Input: part model. Units: mm. Frame: model coordinates. A direction names the side the tool comes from. Give positions to 0.01 mm unless a question says otherwise; leave off trailing zeros. Write each loop counter-clockwise with the first axis right and the second up, starting at its lowest first coordinate (ties: lowest second). Pieces come first, ordered by that corner, then holes. Notation, with made-up numbers: (54.5, 64.25) - (68.5, 64.25) arc R12 cw to (68.5, 78.25) - close; hole circle Ø5 at (30.25, -25). An arc over 180 degrees is marked (long way). Use a Markdown table: item, result. Add a question column.
1. Pin query (flat end, axial travel): pin 1 (2 mm diameter, centred on y = 0, z = -2, fed in from -X); pin 2 (1.2 mm diameter, centred on y = -2, z = -1, fed in from +X); pin 3 (1.5 mm diameter, centred on y = -5.5, z = 3, fed in from +X). Return the tip coordinate at first contact, or that it passes through.
2. Section query D-D, the plane z = 20.75. Return loops of the section in (x, y) (3 decimals), plus the area to 3 significant figures.
3. Section query A-A, the plane y = 0. Count the separate pieces of the cut face and the enclosed holes in it, plus the area to 3 significant figures.
4. Section query B-B, the plane z = 3. Return loops of the section in (x, y) (3 decimals), plus the area to 3 significant figures.
5. Mould query, pull axis X, two halves, no side actions, for faces 1 (the flat face through (-4, -0.1, -4.5)), 2 (the flat face through (0, -8.85, -2)), 3 (the flat face through (0, 7, 1)). Classes: released by +X, released by -X, zero draft, split by the parting line, or undercut.
6. Set-up query: faces 4 (the flat face through (0, 8.85, -2)), 5 (the flat face through (-0.07, 8.04, 6.99)), 6 (the flat face through (-3, 0, 1)). Return all of +Z, -Z, +X, -X, +Y, -Y with unobstructed straight access to the full face (end or side cutting, diameter ignored); none if empty.
7. Section query C-C, the plane x = 0. Return loops of the section in (y, z), plus the area to 3 significant figures.
8. Material intervals for probe 1 along Z at (x, y) = (11.25, 1.25); probe 2 along X at (y, z) = (-1.25, 20); probe 3 along Y at (x, z) = (1.75, 17), sorted ascending.
```python
from build123d import *

# Parameters (mm, degrees)
CROQUIS1_R              = 12.5
SALIENTE_EXTRUIR1_DEPTH = 24
CROQUIS2_W              = 9.3
CROQUIS2_H              = 18
CORTAR_EXTRUIR1_DEPTH   = 18
CROQUIS3_W              = 9
CROQUIS3_H              = 17.7
SALIENTE_EXTRUIR2_DEPTH = 5
CHAFL_N1_SIZE           = 1
CHAFL_N2_SIZE           = 1
CROQUIS4_R              = 2
CORTAR_EXTRUIR2_DEPTH   = 34.963215395
CHAFL_N3_SIZE           = 1
CROQUIS5_W              = 6
CROQUIS5_H              = 14
CORTAR_EXTRUIR3_DEPTH   = 26.228951623
CHAFL_N4_SIZE           = 1.95


with BuildPart() as part:
    # Croquis1 → Saliente-Extruir1 (new body)
    with BuildSketch(Plane.XY):
        Circle(CROQUIS1_R)
    extrude(amount=SALIENTE_EXTRUIR1_DEPTH)

    # Croquis2 → Cortar-Extruir1 (cut)
    with BuildSketch(Plane.XY.offset(24)):
        Rectangle(CROQUIS2_W, CROQUIS2_H)
    extrude(amount=-CORTAR_EXTRUIR1_DEPTH, mode=Mode.SUBTRACT)

    # Croquis3 → Saliente-Extruir2 (add)
    with BuildSketch(Plane(origin=(0, 0, 0), x_dir=(-1, 0, 0), z_dir=(0, 0, -1))):
        Rectangle(CROQUIS3_W, CROQUIS3_H)
    extrude(amount=SALIENTE_EXTRUIR2_DEPTH)

    # Chaflán1
    chafl_n1_edges = [part.edges().sort_by_distance(p)[0] for p in [
        (-4.5, 0, -5),
        (0, 8.85, -5),
        (4.5, 0, -5),
        (0, -8.85, -5),
    ]]
    chamfer(chafl_n1_edges, length=CHAFL_N1_SIZE)

    # Chaflán2
    chafl_n2_edges = [part.edges().sort_by_distance(p)[0] for p in [
        (-12.5, 0, 0),
    ]]
    chamfer(chafl_n2_edges, length=CHAFL_N2_SIZE)

    # Croquis4 → Cortar-Extruir2 (cut, through all)
    with BuildSketch(Plane.XY.offset(24)):
        with Locations((-7.875, 0)):
            Circle(CROQUIS4_R)
        with Locations((7.875, 0)):
            Circle(CROQUIS4_R)
    extrude(amount=-CORTAR_EXTRUIR2_DEPTH, mode=Mode.SUBTRACT)

    # Chaflán3
    chafl_n3_edges = [part.edges().sort_by_distance(p)[0] for p in [
        (-12.5, 0, 24),
    ]]
    chamfer(chafl_n3_edges, length=CHAFL_N3_SIZE)

    # Croquis5 → Cortar-Extruir3 (cut, through all)
    with BuildSketch(Plane.XY.offset(6)):
        Rectangle(CROQUIS5_W, CROQUIS5_H)
    extrude(amount=-CORTAR_EXTRUIR3_DEPTH, mode=Mode.SUBTRACT)

    # Chaflán4
    # the kernel refuses this chamfer: 1.95 mm, written as the material it adds along each edge
    with BuildSketch(Plane(origin=(4.65, 9, 6), x_dir=(0.02749587661058626, 0, 0.9996219169112968), z_dir=(0, -1, 0))) as chafl_n4_piece_1_section:
        Polygon((CHAFL_N4_SIZE * 0.999621916911, CHAFL_N4_SIZE * 0.0274958766106), (-CHAFL_N4_SIZE * 0.0274958766106, CHAFL_N4_SIZE * 0.999621916911), (0, 0), align=None)
    chafl_n4_piece_1 = extrude(amount=18, mode=Mode.PRIVATE)
    chafl_n4_piece_1 = split(chafl_n4_piece_1, bisect_by=Plane(origin=(3, 8, 6.663333333), z_dir=(1, 0, 0)), keep=Keep.TOP, mode=Mode.PRIVATE)
    add(chafl_n4_piece_1)
    with BuildSketch(Plane(origin=(4.65, 9, 6), x_dir=(0.02749587661058626, 0, 0.9996219169112968), z_dir=(0, -1, 0))) as chafl_n4_piece_2_section:
        Polygon((CHAFL_N4_SIZE * 0.999621916911, CHAFL_N4_SIZE * 0.0274958766106), (-CHAFL_N4_SIZE * 0.0274958766106, CHAFL_N4_SIZE * 0.999621916911), (0, 0), align=None)
    chafl_n4_piece_2 = extrude(amount=23.014781827, mode=Mode.PRIVATE)
    chafl_n4_piece_2 = split(chafl_n4_piece_2, bisect_by=Plane(origin=(2.9, 7, 6.1), z_dir=(0, 1, 0)), keep=Keep.TOP, mode=Mode.PRIVATE)
    add(chafl_n4_piece_2)
    with BuildSketch(Plane(origin=(4.65, 14.014781827, 6), x_dir=(0.02749587661058626, 0, 0.9996219169112968), z_dir=(0, -1, 0))) as chafl_n4_piece_3_section:
        Polygon((CHAFL_N4_SIZE * 0.999621916911, CHAFL_N4_SIZE * 0.0274958766106), (-CHAFL_N4_SIZE * 0.0274958766106, CHAFL_N4_SIZE * 0.999621916911), (0, 0), align=None)
    chafl_n4_piece_3 = extrude(amount=23.014781827, mode=Mode.PRIVATE)
    chafl_n4_piece_3 = split(chafl_n4_piece_3, bisect_by=Plane(origin=(2.9, -7, 6.1), z_dir=(0, -1, 0)), keep=Keep.TOP, mode=Mode.PRIVATE)
    add(chafl_n4_piece_3)
    with BuildSketch(Plane(origin=(-4.65, 9, 6), x_dir=(0, 0.02749587661058626, 0.9996219169112968), z_dir=(1, 0, 0)), Plane(origin=(4.65, -9, 6), x_dir=(0, -0.02749587661058626, 0.9996219169112968), z_dir=(-1, 0, 0))) as chafl_n4_piece_4:
        Polygon((CHAFL_N4_SIZE * 0.999621916911, CHAFL_N4_SIZE * 0.0274958766106), (-CHAFL_N4_SIZE * 0.0274958766106, CHAFL_N4_SIZE * 0.999621916911), (0, 0), align=None)
    extrude(amount=9.3)
    with BuildSketch(Plane(origin=(-4.65, -9, 6), x_dir=(-0.02749587661058626, 0, 0.9996219169112968), z_dir=(0, 1, 0))) as chafl_n4_piece_5_section:
        Polygon((CHAFL_N4_SIZE * 0.999621916911, CHAFL_N4_SIZE * 0.0274958766106), (-CHAFL_N4_SIZE * 0.0274958766106, CHAFL_N4_SIZE * 0.999621916911), (0, 0), align=None)
    chafl_n4_piece_5 = extrude(amount=18, mode=Mode.PRIVATE)
    chafl_n4_piece_5 = split(chafl_n4_piece_5, bisect_by=Plane(origin=(-3, -8, 6.663333333), z_dir=(-1, 0, 0)), keep=Keep.TOP, mode=Mode.PRIVATE)
    add(chafl_n4_piece_5)
    with BuildSketch(Plane(origin=(-4.65, -9, 6), x_dir=(-0.02749587661058626, 0, 0.9996219169112968), z_dir=(0, 1, 0))) as chafl_n4_piece_6_section:
        Polygon((CHAFL_N4_SIZE * 0.999621916911, CHAFL_N4_SIZE * 0.0274958766106), (-CHAFL_N4_SIZE * 0.0274958766106, CHAFL_N4_SIZE * 0.999621916911), (0, 0), align=None)
    chafl_n4_piece_6 = extrude(amount=23.014781827, mode=Mode.PRIVATE)
    chafl_n4_piece_6 = split(chafl_n4_piece_6, bisect_by=Plane(origin=(-2.9, -7, 6.1), z_dir=(0, -1, 0)), keep=Keep.TOP, mode=Mode.PRIVATE)
    add(chafl_n4_piece_6)
    with BuildSketch(Plane(origin=(-4.65, -14.014781827, 6), x_dir=(-0.02749587661058626, 0, 0.9996219169112968), z_dir=(0, 1, 0))) as chafl_n4_piece_7_section:
        Polygon((CHAFL_N4_SIZE * 0.999621916911, CHAFL_N4_SIZE * 0.0274958766106), (-CHAFL_N4_SIZE * 0.0274958766106, CHAFL_N4_SIZE * 0.999621916911), (0, 0), align=None)
    chafl_n4_piece_7 = extrude(amount=23.014781827, mode=Mode.PRIVATE)
    chafl_n4_piece_7 = split(chafl_n4_piece_7, bisect_by=Plane(origin=(-2.9, 7, 6.1), z_dir=(0, 1, 0)), keep=Keep.TOP, mode=Mode.PRIVATE)
    add(chafl_n4_piece_7)


solid = part.part
```
Result sheet:
| question | item | result |
|---|---|---|
| 1 | pin 1 | stops at x = -4.5 |
| 1 | pin 2 | stops at x = 4.5 |
| 1 | pin 3 | stops at x = 11.56 |
| 2 | outline | circle Ø25 at (0, 0); hole circle Ø4 at (-7.875, 0); hole (-4.65, -9) - (4.65, -9) - (4.65, 9) - (-4.65, 9) - close; hole circle Ø4 at (7.875, 0) |
| 2 | area | 298 mm² |
| 3 | separate pieces | 4 |
| 3 | enclosed holes | 0 |
| 3 | area | 220 mm² |
| 4 | outline | circle Ø25 at (0, 0); hole circle Ø4 at (-7.875, 0); hole (-3, -7) - (3, -7) - (3, 7) - (-3, 7) - close; hole circle Ø4 at (7.875, 0) |
| 4 | area | 382 mm² |
| 5 | face 1 | released by -X |
| 5 | face 2 | zero draft |
| 5 | face 3 | undercut |
| 6 | face 4 | -Z, +X, -X, +Y |
| 6 | face 5 | +Z |
| 6 | face 6 | +Z, -Z |
| 7 | outline | (-12.5, 1) - (-11.5, 0) - (-8.85, 0) - (-8.85, -4) - (-7.85, -5) - (-7, -5) - (-7, 6) - (-7.05, 6) - (-9, 7.95) - (-9, 24) - (-11.5, 24) - (-12.5, 23) - close; (7, -5) - (7.85, -5) - (8.85, -4) - (8.85, 0) - (11.5, 0) - (12.5, 1) - (12.5, 23) - (11.5, 24) - (9, 24) - (9, 7.95) - (7.05, 6) - (7, 6) - close |
| 7 | area | 211 mm² |
| 8 | probe 1 | z = 0 to 24 |
| 8 | probe 2 | x = -12.44 to -9.44, -6.31 to -4.65, 4.65 to 6.31, 9.44 to 12.44 |
| 8 | probe 3 | y = -12.38 to -9, 9 to 12.38 |
